The listing builds one solid part. Answer for the finished solid, in the listing's coordinates (mm). A direction names the side the tool comes from. Round coordinates to 2 decimals unless told otherwise and drop trailing zeros. Write each loop counter-clockwise with the first axis right and the second up, starting at its lowest first coordinate (ties: lowest second). Pieces come first, ordered by that corner, then holes. Notation, with made-up numbers: (52.25, 66.5) -> (96.25, 66.5) arc R29 ccw to (96.25, 105.5) -> close; hole circle Ø5 at (63, 47.5). An arc over 180 degrees is marked (long way). Write each question's results on one line, items separated by ' | '. Start each with the question number.
```python
from build123d import *

# Parameters (mm, degrees)
F0_R     = 18
F0_R_2   = 13
F1_DEPTH = 2.5
F2_R     = 14.25
F2_R_2   = 13
F3_DEPTH = 5
F4_R     = 2


with BuildPart() as f1:
    # F0 (on Top) → F1 (new body)
    with BuildSketch(Plane.XY):
        Circle(F0_R)
        Circle(F0_R_2, mode=Mode.SUBTRACT)
    extrude(amount=F1_DEPTH)

    # F2 (on face) → F3 (join)
    with BuildSketch(Plane(origin=(0, 0, 0), x_dir=(1, 0, 0), z_dir=(0, 0, -1))):
        Circle(F2_R)
        Circle(F2_R_2, mode=Mode.SUBTRACT)
    extrude(amount=F3_DEPTH)

    # F4
    f4_edges = [f1.edges().sort_by_distance(p)[0] for p in [
        (-18, 0, 2.5),
    ]]
    fillet(f4_edges, radius=F4_R)


solid = f1.part
```
Q1. The part is cut by section C-C, the plane z = -2.25. Write down the section's boundary in (x, y).
Q2. The part is cut by section D-D, the plane z = 1.5. Write down the section's boundary in (x, y), then the cut area to 3 significant figures.
Q3. Determine the mould class of faces 1 (the flat face through (13, -3, -5)), 2 (the cylindrical face through (-10.316, 7.91, -1.197)), 3 (the cylindrical face through (-2.343, 17.847, 0.246)) for opening direction Y: pulls with the +Y half, pulls with the -Y half, needs draft (parallel to the pull), parting line crosses it, or undercut.
Q4. Find the intervals of material crossed by line 1 (Y direction, x = 0, z = -1); line 2 (Z direction, x = 14, y = 4.5), in increasing order.
Q5. The part is cut by section A-A, the plane y = 0. Write down the section's boundary in (x, z), then the cut area to 3 significant figures.
Q6. Each of these flat-tipped pins is pushed along its axis until it touches: pin 1 (11 mm diameter, centred on x = -4, y = 5.5, fed in from -Z); pin 2 (1 mm diameter, centred on x = 3, z = -2, fed in from +Y). Where does it stop, or does it pass through?
Q7. For faces 4 (the cylindrical face through (13.163, 5.458, -2.465)), 5 (the flat face through (-1.3, 13.1, 2.5)), determine the directions among +Z, -Z, +X, -X, +Y, -Y from which every point of the face is accessible in a straight line to the end or side of a thin tool.
Answers follow:
1) outline: circle Ø28.5 at (0, 0); hole circle Ø26 at (0, 0)
2) outline: circle Ø35.46 at (0, 0); hole circle Ø26 at (0, 0) | area: 457 mm^2
3) face 1: needs draft | face 2: undercut | face 3: parting line crosses it
4) line 1: -14.25 to -13, 13 to 14.25 | line 2: 0 to 2.5
5) outline: (-18, 0) -> (-14.25, 0) -> (-14.25, -5) -> (-13, -5) -> (-13, 2.5) -> (-16, 2.5) arc R2 ccw to (-18, 0.5) -> close; (13, -5) -> (14.25, -5) -> (14.25, 0) -> (18, 0) -> (18, 0.5) arc R2 ccw to (16, 2.5) -> (13, 2.5) -> close | area: 35.8 mm^2
6) pin 1: through | pin 2: y = 14.03
7) face 4: -Z | face 5: +Z, +X, -X, +Y, -Y
